Geometry: final body of the model. Coordinates: model frame, mm. A direction names the side the tool comes from. Give positions to 0.01 mm unless a question says otherwise; leave off trailing zeros. Order: outer loops, then holes, each group sorted by start corner. A loop starts at its lowest first (then second) coordinate and runs counter-clockwise, first axis right, second up. Notation, with made-up numbers: (57.25, -40) - (73.25, -40) arc R13 cw to (73.25, -31) - close; hole circle Ø9 at (1, 32). An arc over 180 degrees is marked (long way). Write item = value, one per line. Start each with the question number.
Autodesk Inventor part; units mm, degrees
ref_plane "YZ Plane" through (0, 0, 0) normal (1, 0, 0) x (0, 1, 0)
ref_plane "XZ Plane" through (0, 0, 0) normal (0, 1, 0) x (-1, 0, 0)
ref_plane "XY Plane" through (0, 0, 0) normal (0, 0, 1) x (1, 0, 0)
sketch "Skizze1" plane through (0, 0, 0) normal (0, 0, 1) x (1, 0, 0)
  line L0 (0, 0) -> (-25, 0)
  line L1 (-25, 0) -> (-25, 61)
  line L2 (-25, 61) -> (0, 61)
  line L3 (0, 61) -> (0, 0)
  dimension "d0" = 25
  dimension "d1" = 61
extrude "Extrusion1" add sketch "Skizze1" along normal blind 26
sketch "Skizze2" plane through (0, 0, 26) normal (0, 0, 1) x (1, 0, 0)
  line L0 (-6, 56) -> (-6, 41)
  line L1 (-19, 41) -> (-19, 56)
  line L2 (0, 61) -> (-25, 61)
  line L3 (-25, 61) -> (-25, 0)
  line L4 (0, 0) -> (0, 61)
  line L5 (-6, 20) -> (-6, 5)
  line L6 (-19, 5) -> (-19, 20)
  line L7 (-25, 0) -> (0, 0)
  line L8 (-20, 41) -> (-19, 41)
  line L9 (-5, 41) -> (-5, 20)
  line L10 (-5, 20) -> (-6, 20)
  line L11 (-20, 20) -> (-20, 41)
  line L12 (-6, 41) -> (-5, 41)
  line L13 (-19, 20) -> (-20, 20)
  line L14 (-6, 5) -> (-10.5, 5)
  line L15 (-14.5, 5) -> (-19, 5)
  line L16 (-19, 56) -> (-14.5, 56)
  line L17 (-10.5, 56) -> (-6, 56)
  line L18 (-14.5, 61) -> (-10.5, 61)
  line L19 (-14.5, 0) -> (-10.5, 0)
  line L20 (-14.5, 56) -> (-10.5, 56)
  line L21 (-14.5, 5) -> (-10.5, 5)
  dimension "d4" = 25
  dimension "d5" = 13
  dimension "d6" = 6
  dimension "d7" = 13
  dimension "d8" = 5
  dimension "d9" = 5
  dimension "d10" = 21
extrude "Extrusion2" cut sketch "Skizze2" against normal blind 21 contours L0 L12 L9 L10 L5 L14 L21 L15 L6 L13 L11 L8 L1 L16 L20 L17
sketch "Skizze3" plane through (0, 0, 26) normal (0, 0, 1) x (1, 0, 0)
  line L0 (0, 61) -> (-25, 61)
  line L1 (-19, 56) -> (-6, 56)
  line L2 (-14.5, 61) -> (-10.5, 61)
  line L3 (-10.5, 61) -> (-10.5, 56)
  line L4 (-14.5, 56) -> (-14.5, 61)
  line L5 (-25, 61) -> (-25, 0)
  line L6 (0, 0) -> (0, 61)
  line L7 (-30.0841, 30.5) -> (8.1464, 30.5)
  line L8 (-14.5, 56) -> (-10.5, 56)
  line L9 (-14.5, 5) -> (-14.5, 0)
  line L10 (-10.5, 0) -> (-14.5, 0)
  line L11 (-10.5, 0) -> (-10.5, 5)
  line L12 (-14.5, 5) -> (-10.5, 5)
  point P0 (-19, 5)
  point P1 (-6, 5)
  dimension "d13" = 10.5
  dimension "d14" = 10.5
  dimension "d15" = 4
extrude "Extrusion3" cut sketch "Skizze3" against normal blind 16 contours L3 L1 L4 L0 | L12 L11 L10 L9
ref_plane "Arbeitsebene1" through (-25, 30.5, 0) normal (0, 1, 0) x (1, 0, 0)
sketch "Skizze4" plane through (-25, 30.5, 0) normal (0, 1, 0) x (1, 0, 0)
  line L0 (14.5, -10) -> (10.5, -10)
  line L1 (0, 0) -> (0, -26)
  line L2 (0, -13) -> (-2, -13)
  line L3 (-2, -13) -> (-0.5676, -15.481)
  line L4 (-0.5676, -15.481) -> (0, -16.4641)
  line L5 (0, -13) -> (0, -16.4641)
  line L6 (25, -13) -> (27, -13)
  line L7 (27, -13) -> (25.5676, -15.481)
  line L8 (25.5676, -15.481) -> (25, -16.4641)
  line L9 (25, -13) -> (25, -16.4641)
  line L10 (0, 0) -> (25, 0)
  line L11 (25, -26) -> (14.5, -26)
  dimension "d18" = 2
  dimension "d19" = 60
  dimension "d22" = 13
  dimension "d23" = 9.5359
  dimension "d24" = 26
extrude "Extrusion4" add sketch "Skizze4" along normal mid plane 15
sketch "Skizze6" plane through (0, 0, 0) normal (1, 0, 0) x (0, 0, -1)
  line L0 (-5, 41) -> (-5, 56)
  circle A0 centre (-10, 10) radius 3.5
  line L1 (0, 61) -> (0, 0)
  circle A1 centre (-10, 51) radius 3.5
  line L2 (0, 61) -> (-26, 61)
  line L3 (0, 0) -> (-26, 0)
  dimension "d26" = 7
  dimension "d28" = 7
  dimension "d29" = 10
  dimension "d30" = 10
  dimension "d31" = 10
  dimension "d32" = 10
sketch "Skizze7" plane through (-25, 0, 0) normal (-1, 0, 0) x (0, 0, 1)
  circle A0 centre (10, 51) radius 3.5
  circle A1 centre (10, 10) radius 3.5
  line L0 (0, 61) -> (26, 61)
  line L1 (0, 0) -> (0, 61)
  line L2 (0, 0) -> (26, 0)
  dimension "d33" = 7
  dimension "d34" = 7
  dimension "d35" = 10
  dimension "d36" = 10
  dimension "d37" = 10
  dimension "d38" = 10
extrude "Extrusion5" add sketch "Skizze6" along normal blind 1.8
extrude "Extrusion6" add sketch "Skizze7" along normal blind 1.8
properties part number "valve_body"
Q1. Pull-direction query (X, two-part tool) for faces 5 (the flat face through (-15, 61, 13)), 6 (the flat face through (-10.5, 2, 18)), 7 (the flat face through (-6, 13, 16)), 8 (the flat face through (1.8, 10, 10)); classes: +X half, -X half, draft (parallel to the pull), parting line (faces both ways), or undercut.
Q2. Contact query for flat-ended pins moving along their axis: pin 1 (2 mm diameter, centred on x = -10, y = 16.5, fed in from +Z); pin 2 (4.5 mm diameter, centred on y = 51.5, z = 14.5, fed in from -X); pin 3 (3 mm diameter, centred on y = 13.5, z = 15, fed in from +X). Output: stop coordinate, or through.
Q3. Material intervals for line 1 along Y through (x, z) = (-10, 21.25); line 2 along X through (y, z) = (4, 22.5); line 3 along X through (y, z) = (48, 13.75), sorted ascending. Write a range as from..to.
Q4. Section C-C, the plane y = 39.5. Return the cut outline in (x, z), then the cut area to 3 significant figures.
Q5. Section A-A, the plane z = 20.25. Return the cut outline in (x, y).
Q6. Section B-B, the plane y = 24. Return the cut outline in (x, z), then the cut area to 3 significant figures.
Q7. Set-up query: faces 1 (the flat face through (-5, 31, 16)), 2 (the cylindrical face through (-25.887, 9.846, 6.503)), 3 (the flat face through (-13, 3, 10)), 4 (the cylindrical face through (0.89, 47.53, 10.46)). Return all of +Z, -Z, +X, -X, +Y, -Y with unobstructed straight access to the full face (end or side cutting, diameter ignored); none if empty.
The answers:
q1.face_5 = draft
q1.face_6 = undercut
q1.face_7 = undercut
q1.face_8 = +X half
q2.pin_1 = 5
q2.pin_2 = -26.8
q2.pin_3 = 0
q3.line_1 = 0..5, 56..61
q3.line_2 = -25..-14.5, -10.5..0
q3.line_3 = -25..-19, -6..0
q4.outline = (-25, 0) - (0, 0) - (0, 26) - (-5, 26) - (-5, 5) - (-20, 5) - (-20, 26) - (-25, 26) - close
q4.area = 335 mm²
q5.outline = (-25, 0) - (-14.5, 0) - (-14.5, 5) - (-19, 5) - (-19, 20) - (-20, 20) - (-20, 41) - (-19, 41) - (-19, 56) - (-14.5, 56) - (-14.5, 61) - (-25, 61) - close; (-10.5, 0) - (0, 0) - (0, 61) - (-10.5, 61) - (-10.5, 56) - (-6, 56) - (-6, 41) - (-5, 41) - (-5, 20) - (-6, 20) - (-6, 5) - (-10.5, 5) - close
q6.outline = (-27, 13) - (-25, 13) - (-25, 0) - (0, 0) - (0, 13) - (2, 13) - (0.57, 15.48) - (0, 16.46) - (0, 26) - (-5, 26) - (-5, 5) - (-20, 5) - (-20, 26) - (-25, 26) - (-25, 16.46) - (-25.57, 15.48) - close
q6.area = 342 mm²
q7.face_1 = +Z
q7.face_2 = -X
q7.face_3 = +Z, +Y, -Y
q7.face_4 = +X
